Geometry check sheet. Reference: the model listing, model coordinates, mm. Round coordinates to 2 decimals unless told otherwise and drop trailing zeros. Loops run counter-clockwise (first coordinate to the right, second up) from the corner with the lowest first, then second, coordinate; pieces in that order, holes last.
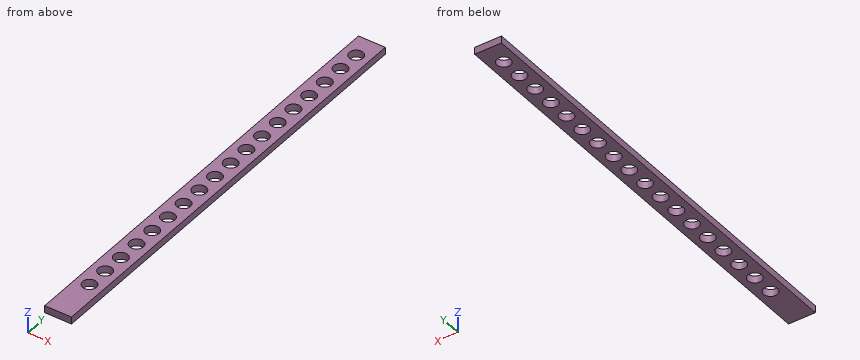
```python
from build123d import *

# Parameters (mm, degrees)
SKETCH1_W           = 6
SKETCH1_H           = 100
MAINBODY_DEPTH      = 1.5875
PEGHOLE_REACH       = 52.115
SKETCH2_R           = 1.55
LPATTERN1_COUNT     = 9
LPATTERN1_PITCH     = 5
LPATTERN2_OUTLINE_R = 1.55
LPATTERN2_DEPTH     = 1.5875


# Read off the part's stored shape, not the designer's step: LPattern2
with BuildPart() as part:
    # Sketch1 → MainBody (new body)
    with BuildSketch(Plane.XY):
        Rectangle(SKETCH1_W, SKETCH1_H)
    extrude(amount=MAINBODY_DEPTH)

    # Sketch2 → PegHole (cut, up to next)
    with BuildSketch(Plane.XY.offset(1.5875), mode=Mode.PRIVATE) as peghole_sk1:
        Circle(SKETCH2_R)
    peghole_tool1 = extrude(peghole_sk1.sketch, amount=-PEGHOLE_REACH, mode=Mode.PRIVATE) & part.part
    peghole = peghole_tool1.solids().sort_by_distance((0, 0, 1.5875))[0]
    add(peghole, mode=Mode.SUBTRACT)

    # LPattern1: PegHole ×9
    with Locations(*[(0, -i * LPATTERN1_PITCH, 0) for i in range(1, LPATTERN1_COUNT)]):
        add(peghole, mode=Mode.SUBTRACT)

    # LPattern2 outline → LPattern2 (cut)
    with BuildSketch(Plane.XY):
        with Locations((0, 5)):
            Circle(LPATTERN2_OUTLINE_R)
        with Locations((0, 10)):
            Circle(LPATTERN2_OUTLINE_R)
        with Locations((0, 15)):
            Circle(LPATTERN2_OUTLINE_R)
        with Locations((0, 20)):
            Circle(LPATTERN2_OUTLINE_R)
        with Locations((0, 25)):
            Circle(LPATTERN2_OUTLINE_R)
        with Locations((0, 30)):
            Circle(LPATTERN2_OUTLINE_R)
        with Locations((0, 35)):
            Circle(LPATTERN2_OUTLINE_R)
        with Locations((0, 40)):
            Circle(LPATTERN2_OUTLINE_R)
        with Locations((0, 45)):
            Circle(LPATTERN2_OUTLINE_R)
    extrude(amount=LPATTERN2_DEPTH, mode=Mode.SUBTRACT)


solid = part.part
```
1) Sectioned sample at A-A, the plane y = 15. Record the cut outline in (x, z), then the cut area to 3 significant figures.
Report:
outline: (-3, 0) - (-1.55, 0) - (-1.55, 1.59) - (-3, 1.59) - close; (1.55, 0) - (3, 0) - (3, 1.59) - (1.55, 1.59) - close
area: 4.60 mm2
2) Sectioned sample at B-B, the plane z = 0.55. State how many separate pieces and enclosed holes the cut face has, then the cut area to 3 significant figures.
Report:
separate pieces: 1
enclosed holes: 18
area: 464 mm2
3) Scan lines: line 1 along X through (y, z) = (9.5, 0.9); line 2 along X through (y, z) = (21, 0.85). Record each from-to range of solid material in increasing order.
Report:
line 1: x = -3 to -1.47, 1.47 to 3
line 2: x = -3 to -1.18, 1.18 to 3
